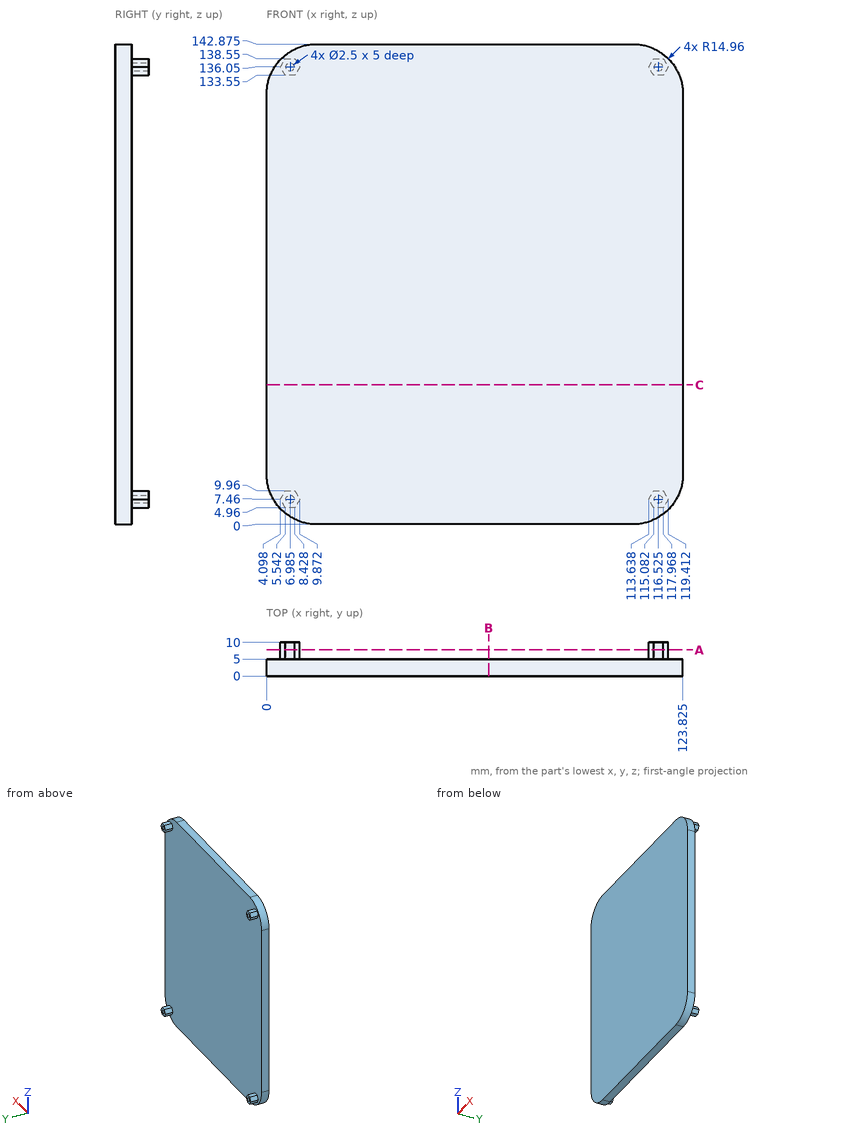
Geometry check sheet. Reference: drawing and pictorial views, mm from the part's lowest x, y, z. Coordinates: 2 decimals unless noted, no trailing zeros. Loops run counter-clockwise (first coordinate to the right, second up) from the corner with the lowest first, then second, coordinate; pieces in that order, holes last. Notation, with made-up numbers: (36.5, 19.5) - (67.5, 19.5) arc R22 cw to (67.5, 50.5) - close; hole circle Ø8 at (20, 57.5). An arc over 180 degrees is marked (long way). Return JSON: item names as keys, results as strings.
1. Section check B-B, the plane x = 66. Record the boundary of the cut face in (y, z) (1 decimal).
Established:
{"outline": "(0, 0) - (5, 0) - (5, 142.9) - (0, 142.9) - close"}
2. Section check C-C, the plane z = 41.5. Record the boundary of the cut face in (x, y) (1 decimal).
Established:
{"outline": "(0, 0) - (123.8, 0) - (123.8, 5) - (0, 5) - close"}
3. Section check A-A, the plane y = 7.75. Count the separate pieces of the cut face and the enclosed holes in it.
Established:
{"separate pieces": "4", "enclosed holes": "4"}
4. Go/stop test with flat-tipped pins: pin 1 (1.4 mm diameter, centred on x = 7.5, y = 6.5, fed in from -Z); pin 2 (1.2 mm diameter, centred on x = 116, z = 7.5, fed in from +Y); pin 3 (0.9 mm diameter, centred on x = 6.5, y = 8, fed in from +Z). Record where each tip stops, or that it passes through.
Established:
{"pin 1": "stops at z = 4.96", "pin 2": "stops at y = 5", "pin 3": "stops at z = 138.55"}
5. Thickness scan on L1, parallel to X at y = 7.05, z = 136.05 (1 decimal); L2, parallel to Y at x = 78, z = 90; L3, parallel to X at y = 9.25, z = 8.5. Record the ranges inside material, lowest first.
Established:
{"L1": "x = 4.1 to 5.7, 8.2 to 9.9, 113.6 to 115.3, 117.8 to 119.4", "L2": "y = 0 to 5", "L3": "x = 4.7 to 6.29, 7.68 to 9.27, 114.24 to 115.83, 117.22 to 118.81"}
